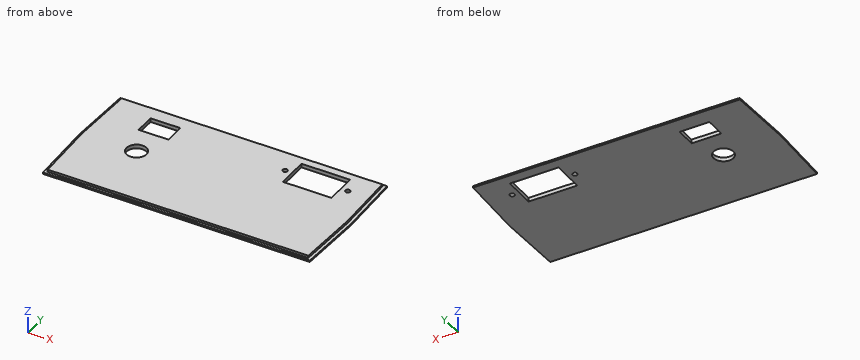
```python
from build123d import *

# Parameters (mm, degrees)
BOSS_EXTRUDE1_DEPTH = 1
BOSS_EXTRUDE2_DEPTH = 1.5
CUT_EXTRUDE1_REACH  = 98.19
SKETCH3_R           = 1.5
SKETCH3_R_2         = 6.35
SKETCH3_W           = 31
SKETCH3_H           = 20.4
SKETCH3_W_2         = 19
SKETCH3_H_2         = 13


with BuildPart() as part:
    # Sketch1 → Boss-Extrude1 (new body)
    with BuildSketch(Plane.XY):
        Polygon((-85, 42), (85, 42), (86.5, 0), (85, -42), (-85, -42), (-86.5, 0), align=None)
    extrude(amount=BOSS_EXTRUDE1_DEPTH)

    # Sketch2 → Boss-Extrude2 (add)
    with BuildSketch(Plane.XY.offset(1)):
        Polygon((-83, 40.25), (83, 40.25), (84.5, 0), (83, -40.25), (-83, -40.25), (-84.5, 0), align=None)
    extrude(amount=BOSS_EXTRUDE2_DEPTH)

    # Sketch3 → Cut-Extrude1 (cut, up to next)
    with BuildSketch(Plane(origin=(0, 0, 0), x_dir=(-1, 0, 0), z_dir=(0, 0, -1)), mode=Mode.PRIVATE) as cut_extrude1_sk1:
        with Locations((-70, 25)):
            Circle(SKETCH3_R)
    cut_extrude1_tool1 = extrude(cut_extrude1_sk1.sketch, amount=-CUT_EXTRUDE1_REACH, mode=Mode.PRIVATE) & part.part
    # Sketch3 → Cut-Extrude1 (cut, up to next)
    with BuildSketch(Plane(origin=(0, 0, 0), x_dir=(-1, 0, 0), z_dir=(0, 0, -1)), mode=Mode.PRIVATE) as cut_extrude1_sk2:
        with Locations((-30, 25)):
            Circle(SKETCH3_R)
    cut_extrude1_tool2 = extrude(cut_extrude1_sk2.sketch, amount=-CUT_EXTRUDE1_REACH, mode=Mode.PRIVATE) & part.part
    # Sketch3 → Cut-Extrude1 (cut, up to next)
    with BuildSketch(Plane(origin=(0, 0, 0), x_dir=(-1, 0, 0), z_dir=(0, 0, -1)), mode=Mode.PRIVATE) as cut_extrude1_sk3:
        with Locations((50, 0)):
            Circle(SKETCH3_R_2)
    cut_extrude1_tool3 = extrude(cut_extrude1_sk3.sketch, amount=-CUT_EXTRUDE1_REACH, mode=Mode.PRIVATE) & part.part
    # Sketch3 → Cut-Extrude1 (cut, up to next)
    with BuildSketch(Plane(origin=(0, 0, 0), x_dir=(-1, 0, 0), z_dir=(0, 0, -1)), mode=Mode.PRIVATE) as cut_extrude1_sk4:
        with Locations((-50, 25)):
            Rectangle(SKETCH3_W, SKETCH3_H)
    cut_extrude1_tool4 = extrude(cut_extrude1_sk4.sketch, amount=-CUT_EXTRUDE1_REACH, mode=Mode.PRIVATE) & part.part
    # Sketch3 → Cut-Extrude1 (cut, up to next)
    with BuildSketch(Plane(origin=(0, 0, 0), x_dir=(-1, 0, 0), z_dir=(0, 0, -1)), mode=Mode.PRIVATE) as cut_extrude1_sk5:
        with Locations((50, 25)):
            Rectangle(SKETCH3_W_2, SKETCH3_H_2)
    cut_extrude1_tool5 = extrude(cut_extrude1_sk5.sketch, amount=-CUT_EXTRUDE1_REACH, mode=Mode.PRIVATE) & part.part
    add(cut_extrude1_tool1.solids().sort_by_distance((70, 25, 0))[0], mode=Mode.SUBTRACT)
    add(cut_extrude1_tool2.solids().sort_by_distance((30, 25, 0))[0], mode=Mode.SUBTRACT)
    add(cut_extrude1_tool3.solids().sort_by_distance((-50, 0, 0))[0], mode=Mode.SUBTRACT)
    add(cut_extrude1_tool4.solids().sort_by_distance((50, 25, 0))[0], mode=Mode.SUBTRACT)
    add(cut_extrude1_tool5.solids().sort_by_distance((-50, 25, 0))[0], mode=Mode.SUBTRACT)


solid = part.part
```
Build history of the part. All positions in model axes, mm. Coordinates: 2 decimals unless noted, no trailing zeros. Order: outer loops, then holes, each group sorted by start corner. A loop starts at its lowest first (then second) coordinate and runs counter-clockwise, first axis right, second up. Notation, with made-up numbers: M 3.5,42 L 29.5,42 A8 cw 29.5,51 Z; hole C 28.5,-21 d5. An arc over 180 degrees is marked long. One line per question, with ' | ' between items. Start each with the question number.
1. Cut at C-C (z = 1.9). Write the cut outline in (x, y), plus the area to 3 significant figures.
2. Cut at A-A (x = 54). Write the cut outline in (y, z), plus the area to 3 significant figures.
3. Wall check: line 1 along X through (y, z) = (22.5, 2); line 2 along X through (y, z) = (0.5, 0.2); line 3 along X through (y, z) = (30.5, 1.7). Give the ranges that are in metal, low to high. Write a range as [from, to].
4. Flat gauge pins, fed straight in: P1, Ø1.2, axis at y = 22, z = 1.5, coming from the +X side; P2, Ø1.2, axis at x = -22.5, z = 2, coming from the -Y side; P3, Ø0.8, axis at y = 23.5, z = 1.5, coming from the -X side. Where does each tip first touch, or does it go through?
5. Cut at B-B (x = -50). Write the cut outline in (y, z), plus the area to 4 significant figures.
6. Cut at D-D (y = -4.5). Write the cut outline in (x, z).
The answers:
1) outline: M -84.5,0 L -83,-40.25 L 83,-40.25 L 84.5,0 L 83,40.25 L -83,40.25 Z; hole M -59.5,18.5 L -40.5,18.5 L -40.5,31.5 L -59.5,31.5 Z; hole C -50,0 d12.7; hole C 30,25 d3; hole M 34.5,14.8 L 65.5,14.8 L 65.5,35.2 L 34.5,35.2 Z; hole C 70,25 d3 | area: 12,500 mm2
2) outline: M -42,0 L 14.8,0 L 14.8,2.5 L -40.25,2.5 L -40.25,1 L -42,1 Z; M 35.2,0 L 42,0 L 42,1 L 40.25,1 L 40.25,2.5 L 35.2,2.5 Z | area: 154 mm2
3) line 1: x = [-83.66, -59.5], [-40.5, 34.5], [65.5, 83.66] | line 2: x = [-86.48, -56.33], [-43.67, 86.48] | line 3: x = [-83.36, -59.5], [-40.5, 34.5], [65.5, 83.36]
4) P1: stops at x = 85.73 | P2: stops at y = -40.25 | P3: stops at x = -83.64
5) outline: M -42,0 L -6.35,0 L -6.35,2.5 L -40.25,2.5 L -40.25,1 L -42,1 Z; M 6.35,0 L 18.5,0 L 18.5,2.5 L 6.35,2.5 Z; M 31.5,0 L 42,0 L 42,1 L 40.25,1 L 40.25,2.5 L 31.5,2.5 Z | area: 140.5 mm2
6) outline: M -86.34,0 L -54.48,0 L -54.48,2.5 L -84.33,2.5 L -84.33,1 L -86.34,1 Z; M -45.52,0 L 86.34,0 L 86.34,1 L 84.33,1 L 84.33,2.5 L -45.52,2.5 Z
